Here's how the part is built. I have some questions about the finished solid (model axes, mm). Face numbers are marked on the shaded views. A direction names the side the tool comes from. Coordinates: 2 decimals unless noted, no trailing zeros. Order: outer loops, then holes, each group sorted by start corner. A loop starts at its lowest first (then second) coordinate and runs counter-clockwise, first axis right, second up. Notation, with made-up numbers: (-33.75, 11) - (-11.75, 11) arc R20 ccw to (-11.75, 28) - close; hole circle Ø8 at (71, 84.5). An arc over 180 degrees is marked (long way). Answer as CSV lines item,"result". Start each with the question number.
Q1. Thinking about a two-plate mould opening in X: for the marked faces 1, 2 and 3, which applies, released by +X, released by -X, zero draft, split by the parting line, or undercut?
Q2. Suppose I cut it at B-B (y = -42). Please give me the cut outline in (x, z), then the cut area to 3 significant figures.
Q3. Suppose I cut it at D-D (z = 20.5). Please give me the cut outline in (x, y) (1 decimal).
Q4. I need wall thicknesses on line 1 (Z direction, x = 0, y = -31.25); line 2 (Y direction, x = 0, z = 21.75); line 3 (X direction, y = -33.5, z = 12.7). Which ranges of each line are inside material? Lowest first, please.
Q5. For the marked faces 4, 5 and 6, which set-ups out of +Z, -Z, +X, -X, +Y, -Y let a thin tool reach every point of the face, with its end or its side?
Q6. Suppose I cut it at C-C (x = 11.5). Please give me the cut outline in (y, z), then the cut area to 3 significant figures.
Q7. For pin 1 Ø3 at (y, z) = (-13, 17) entering from -X; pin 2 Ø12 at (y, z) = (-9.5, 4.5) entering from +X; pin 3 Ø2 at (y, z) = (-12, 11) entering from -X, each with a flat end and sliding along its axis, tell me the tip position at first contact or that it passes through.
Q8. Suppose I cut it at A-A (y = -81.5). Please give me the cut outline in (x, z), then the cut area to 3 significant figures.
from build123d import *

# Parameters (mm, degrees)
F1_DEPTH = 25.4
F3_D     = 10.0838
F3_DEPTH = 19.05
F3_TIP   = 3.0294791551
F5_D     = 6.477
F5_DEPTH = 14.2748
F5_TIP   = 1.9458871147
F6_SIZE  = 1.27


with BuildPart() as f1:
    # F0 (on Top) → F1 (new body)
    with BuildSketch(Plane.XY):
        with BuildLine():
            Line((-12.8905, 0), (-18.9865, 0))
            Line((-18.9865, 0), (-36.5125, -25.4))
            Line((-36.5125, -25.4), (-36.5125, -88.9))
            Line((-36.5125, -88.9), (-7.9375, -88.9))
            Line((-7.9375, -88.9), (-7.9375, -76.2127))
            ThreePointArc((-7.9375, -76.2127), (0, -68.2752), (7.9375, -76.2127))
            Line((7.9375, -76.2127), (7.9375, -88.9))
            Line((7.9375, -88.9), (36.5125, -88.9))
            Line((36.5125, -88.9), (36.5125, -25.4))
            Line((36.5125, -25.4), (18.9865, 0))
            Line((18.9865, 0), (12.8905, 0))
            Line((12.8905, 0), (12.8905, -25.4))
            Line((12.8905, -25.4), (-12.8905, -25.4))
            Line((-12.8905, -25.4), (-12.8905, 0))
        make_face()
    extrude(amount=F1_DEPTH)

    # F3
    with Locations(Plane(origin=(0, -25.4, 0), x_dir=(-1, 0, 0), z_dir=(0, 1, 0))):
        with Locations((0, 12.7)):
            Hole(F3_D / 2, depth=F3_DEPTH)
            with Locations((0, 0, -(F3_DEPTH + F3_TIP / 2))):  # 118° drill point
                Cone(0, F3_D / 2, F3_TIP, mode=Mode.SUBTRACT)

    # F5
    with Locations(Plane.XY.offset(25.4)):
        with Locations((0, -61.9252)):
            Hole(F5_D / 2, depth=F5_DEPTH)
            with Locations((0, 0, -(F5_DEPTH + F5_TIP / 2))):  # 118° drill point
                Cone(0, F5_D / 2, F5_TIP, mode=Mode.SUBTRACT)

    # F6
    f6_edges = [f1.edges().sort_by_distance(p)[0] for p in [
        (-22.225, -88.9, 25.4),
        (-15.9385, 0, 25.4),
        (-27.7495, -12.7, 25.4),
        (-36.5125, -57.15, 25.4),
        (15.9385, 0, 25.4),
        (27.7495, -12.7, 25.4),
        (36.5125, -57.15, 25.4),
        (22.225, -88.9, 25.4),
    ]]
    chamfer(f6_edges, length=F6_SIZE)


solid = f1.part
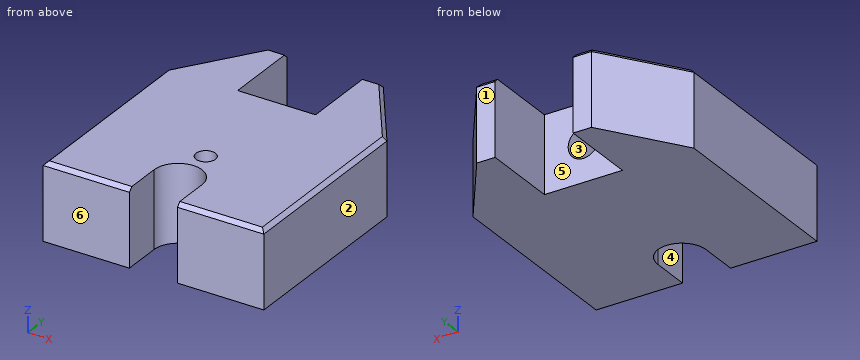
Here are the results:
1,face 1,"zero draft"
1,face 2,"released by +X"
1,face 3,"undercut"
2,outline,"(-36.51, 0) - (36.51, 0) - (36.51, 24.13) - (35.24, 25.4) - (-35.24, 25.4) - (-36.51, 24.13) - close; hole circle Ø10.08 at (0, 12.7)"
2,area,"1,770 mm²"
3,outline,"(-36.5, -88.9) - (-7.9, -88.9) - (-7.9, -76.2) arc R7.9 cw to (7.9, -76.2) - (7.9, -88.9) - (36.5, -88.9) - (36.5, -25.4) - (19, 0) - (12.9, 0) - (12.9, -25.4) - (-12.9, -25.4) - (-12.9, 0) - (-19, 0) - (-36.5, -25.4) - close; hole circle Ø6.5 at (0, -61.9)"
4,line 1,"z = 0 to 7.66, 17.74 to 25.4"
4,line 2,"y = -68.28 to -65.16, -58.69 to -25.4"
4,line 3,"x = -36.51 to -5.04, 5.04 to 36.51"
5,face 4,"+Z, -Z, -Y"
5,face 5,"+Z, -Z, +Y"
5,face 6,"+Z, -Z, +X, -X, -Y"
6,outline,"(-88.9, 0) - (-25.4, 0) - (-25.4, 25.4) - (-87.63, 25.4) - (-88.9, 24.13) - close"
6,area,"1,610 mm²"
7,pin 1,"stops at x = -28.99"
7,pin 2,"stops at x = 29.68"
7,pin 3,"stops at x = -27.96"
8,outline,"(-36.51, 0) - (-7.94, 0) - (-7.94, 25.4) - (-35.24, 25.4) - (-36.51, 24.13) - close; (7.94, 0) - (36.51, 0) - (36.51, 24.13) - (35.24, 25.4) - (7.94, 25.4) - close"
8,area,"1,450 mm²"
